Autodesk Inventor part; units mm, degrees
ref_plane "YZ Plane" through (0, 0, 0) normal (1, 0, 0) x (0, 1, 0)
ref_plane "XZ Plane" through (0, 0, 0) normal (0, 1, 0) x (-1, 0, 0)
ref_plane "XY Plane" through (0, 0, 0) normal (0, 0, 1) x (1, 0, 0)
sketch "Sketch1" plane through (0, 0, 0) normal (0, 0, 1) x (1, 0, 0)
  line L0 (0, 0) -> (3.175, 0)
  line L1 (3.175, 0) -> (3.175, 50.8)
  line L2 (3.175, 50.8) -> (0, 50.8)
  line L3 (0, 50.8) -> (0, 0)
  line L4 (0, 0) -> (50.8, 0)
  line L5 (50.8, 0) -> (50.8, 3.175)
  line L6 (50.8, 3.175) -> (0, 3.175)
  line L7 (0, 3.175) -> (0, 0)
  dimension "d0" = 3.175
  dimension "d1" = 50.8
  dimension "d2" = 50.8
  dimension "d3" = 3.175
extrude "Extrusion1" add sketch "Sketch1" along normal blind 25.4
sketch "Sketch2" plane through (3.175, 3.175, 0) normal (1, 0, 0) x (0, 0, -1)
  line L0 (0, 47.625) -> (-25.4, 47.625)
  line L1 (-12.7, 47.625) -> (-12.7, 22.225)
  circle A0 centre (-12.7, 34.925) radius 7.9057
  point P0 (0, -3.175)
  dimension "d6" = 25.4
  dimension "d7" = 15.8115
extrude "Extrusion2" cut sketch "Sketch2" against normal blind 25.4
sketch "Sketch3" plane through (3.175, 3.175, 0) normal (0, 1, 0) x (1, 0, 0)
  line L0 (47.625, 0) -> (47.625, -25.4) construction
  line L1 (47.625, -12.7) -> (34.925, -12.7) construction
  line L2 (47.625, -12.7) -> (60.325, -12.7) construction
  circle A0 centre (34.925, -12.7) radius 2.5797
  line L3 (34.925, -12.7) -> (9.525, -12.7) construction
  circle A1 centre (9.525, -12.7) radius 2.5797
  point P0 (-3.175, 0)
  dimension "d10" = 12.7
  dimension "d11" = 180
  dimension "d12" = 5.1594
  dimension "d15" = 25.4
extrude "Extrusion4" cut sketch "Sketch3" against normal blind 25.4
properties part number "Piston bracket"
The listing builds one solid part. Answer for the finished solid, in the listing's coordinates (mm). A direction names the side the tool comes from. Give positions to 0.01 mm unless a question says otherwise; leave off trailing zeros. Write each loop counter-clockwise with the first axis right and the second up, starting at its lowest first coordinate (ties: lowest second). Pieces come first, ordered by that corner, then holes. Notation, with made-up numbers: (-18, 4) - (-7, 4) arc R29 cw to (-7, 39) - close; hole circle Ø6 at (55.25, 89). An arc over 180 degrees is marked (long way). Use one line per item in the form item = value. Start each with the question number.
1) Flat-ended cylindrical pins translate along their axes: pin 1 Ø8 at (x, z) = (35, 10.5) entering from +Y (3 decimals); pin 2 Ø6 at (x, z) = (12.7, 12.7) entering from -Y; pin 3 Ø10 at (y, z) = (20.5, 7) entering from +X (3 decimals). Find the tip coordinate at first contact, or state that the pin passes through.
2) The mould has two halves that part along Z. Classify faces 1 (the face through (27, 3.175, 13)), 2 (the face through (3, 14, 25.4)), 3 (the face through (3, 14, 0)), 4 (the face through (1.61, 45.94, 13.73)): pulls with the +Z half, pulls with the -Z half, needs draft (parallel to the pull), parting line crosses it, or undercut.
3) Find section A-A on y = 38.1. Determine the outline of the cut face in (x, z) (3 decimals), plus the area to 3 significant figures.
4) Consider line 1 along X through (y, z) = (2.4, 12.7); line 2 along Y through (x, z) = (1.15, 12.7); line 3 along Z through (x, y) = (38.1, 1.25). Determine where each line is inside the solid, lowest interval first. Write a range as from..to.
5) A tool of negligible diameter and unlimited length cuts with its end or side. For faces 5 (the face through (3.175, 27, 13)), 6 (the face through (0, 26, 13)), from which of +Z, -Z, +X, -X, +Y, -Y can it reach the whole face along a straight path? Write none if from no direction.
6) Find section C-C on z = 17.5. Determine the outline of the cut face in (x, y) (3 decimals), plus the area to 3 significant figures.
7) Find section D-D on y = 24. Determine the outline of the cut face in (x, z) (3 decimals).
8) Find section B-B on x = 12.7. Determine the outline of the cut face in (y, z) (3 decimals).
Geometry results:
q1.pin_1 = 3.175
q1.pin_2 = 0
q1.pin_3 = 3.175
q2.face_1 = needs draft
q2.face_2 = pulls with the +Z half
q2.face_3 = pulls with the -Z half
q2.face_4 = undercut
q3.outline = (0, 0) - (3.175, 0) - (3.175, 4.794) - (0, 4.794) - close; (0, 20.606) - (3.175, 20.606) - (3.175, 25.4) - (0, 25.4) - close
q3.area = 30.4 mm2
q4.line_1 = 0..10.12, 15.28..35.52, 40.68..50.8
q4.line_2 = 0..30.19, 46.01..50.8
q4.line_3 = 0..10.12, 15.28..25.4
q5.face_5 = +Z, -Z, +X, +Y
q5.face_6 = +Z, -Z, -X, +Y, -Y
q6.outline = (0, 0) - (50.8, 0) - (50.8, 3.175) - (3.175, 3.175) - (3.175, 31.818) - (0, 31.818) - close; (0, 44.382) - (3.175, 44.382) - (3.175, 50.8) - (0, 50.8) - close
q6.area = 273 mm2
q7.outline = (0, 0) - (3.175, 0) - (3.175, 25.4) - (0, 25.4) - close
q8.outline = (0, 0) - (3.175, 0) - (3.175, 10.12) - (0, 10.12) - close; (0, 15.28) - (3.175, 15.28) - (3.175, 25.4) - (0, 25.4) - close
